Read the model definition and answer for the solid it produces. Units are mm, in the model's axes. Face numbers are marked on the shaded views. A direction names the side the tool comes from. Coordinates: 2 decimals unless noted, no trailing zeros. Order: outer loops, then holes, each group sorted by start corner. A loop starts at its lowest first (then second) coordinate and runs counter-clockwise, first axis right, second up. Notation, with made-up numbers: (61, 10.5) -> (112, 10.5) arc R28 ccw to (112, 38.5) -> close; hole circle Ø8 at (-37.5, 45). An arc over 180 degrees is marked (long way). Answer as a JSON object with one key per item and string values. Group by question number.
1) Determine the mould class of the marked faces 1, 2 and 3 for opening direction Z: released by +Z, released by -Z, zero draft, split by the parting line, or undercut.
2) A tool of negligible diameter and unlimited length cuts with its end or side. For the marked faces 4, 5, 6, 7 and 8, from which of +Z, -Z, +X, -X, +Y, -Y can it reach the whole face along a straight path? Write none if from no direction.
3) Section C-C on x = 104.5 is taken. Count the separate pieces of the cut face and the enclosed holes in it, and give its area (3 significant figures).
4) Section D-D on z = 31.5 is taken. Determine the outline of the cut face in (x, y), and give its area (3 significant figures).
5) Given pin 1 (3 mm diameter, centred on x = 87.5, z = 10.5, fed in from +Y); pin 2 (12 mm diameter, centred on y = 79, z = 19, fed in from -X); pin 3 (16.5 mm diameter, centred on y = 18.5, z = 22, fed in from -X), each flat-ended and moving along its own axis, determine where each tip first touches the part or whether it passes through.
6) Consider L1, parallel to Z at x = 105.5, y = 70.5; L2, parallel to Y at x = 118, z = 28.5; L3, parallel to Z at x = 96.5, y = 57. Determine where each line is inside the solid, lowest interval first.
7) Section B-B on y = 25 is taken. Determine the outline of the cut face in (x, z), and give its area (3 significant figures).
8) Section A-A on z = 7 is taken. Determine the outline of the cut face in (x, y), and give its area (3 significant figures).
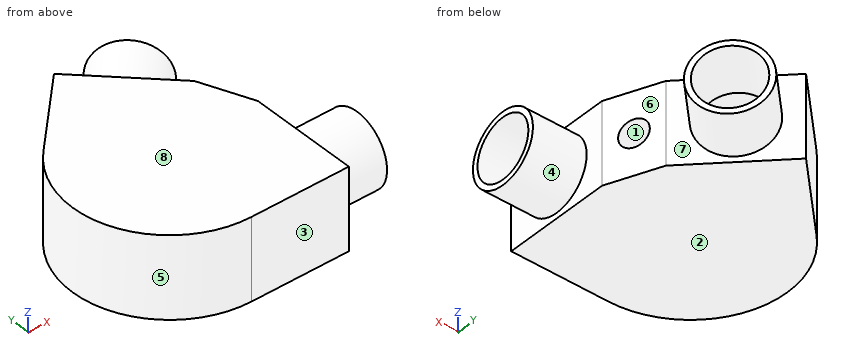
from build123d import *

# Parameters (mm, degrees)
F1_DEPTH = 38
F2_R     = 16.5
F3_DEPTH = 25
F4_R     = 45
F5_R     = 16.5
F6_DEPTH = 25
F7_R     = 6.35
F8_DEPTH = 50
F9_T     = -2.5


with BuildPart() as f1:
    # F0 (on Top) → F1 (new body)
    with BuildSketch(Plane.XY):
        Polygon((85.0829000017, 108.8944443027), (-23.811544301, 0), (130.188455699, 0), (130.188455699, 50), (120.4382390611, 73.5391052434), align=None)
    extrude(amount=F1_DEPTH)

    # F2 (on face) → F3 (join)
    with BuildSketch(Plane.YZ.offset(130.188455699)):
        with Locations((25, 19)):
            Circle(F2_R)
    extrude(amount=F3_DEPTH)

    # F4
    f4_edges = [f1.edges().sort_by_distance(p)[0] for p in [
        (-23.811544, 0, 19),
    ]]
    fillet(f4_edges, radius=F4_R)

    # F5 (on face) → F6 (join)
    with BuildSketch(Plane(origin=(96.9886721522, 96.9886721522, 0), x_dir=(-0.7071067812, 0.7071067812, 0), z_dir=(0.7071067812, 0.7071067812, 0))):
        with Locations((-8.1626955542, 19)):
            Circle(F5_R)
    extrude(amount=F6_DEPTH)

    # F7 (on face) → F8 (cut)
    with BuildSketch(Plane(origin=(128.8004673077, 53.3509003988, 0), x_dir=(-0.3826834324, 0.9238795325, 0), z_dir=(0.9238795325, 0.3826834324, 0))):
        with Locations((9.112283503, 19)):
            Circle(F7_R)
    extrude(amount=-F8_DEPTH, mode=Mode.SUBTRACT)

    # F9
    f9_openings = [f1.faces().sort_by_distance(p)[0] for p in [
        (155.188456, 25, 19),
        (120.438239, 108.894444, 19),
    ]]
    offset(amount=F9_T, openings=f9_openings, kind=Kind.INTERSECTION)


solid = f1.part
Worked answers:
{
 "1": {"face 1": "undercut", "face 2": "released by -Z", "face 3": "zero draft"},
 "2": {"face 4": "+X", "face 5": "+Z, -Z, -X", "face 6": "+Z, -Z, +X", "face 7": "none", "face 8": "+Z, +X, -X, +Y, -Y"},
 "3": {"separate pieces": "2", "enclosed holes": "2", "area": "867 mm²"},
 "4": {"outline": "(53.01, 76.82) arc R45 ccw to (84.83, 0) -> (130.19, 0) -> (130.19, 14.23) -> (155.19, 14.23) -> (155.19, 18.7) -> (127.69, 18.7) -> (127.69, 2.5) -> (84.83, 2.5) arc R42.5 cw to (54.78, 75.05) -> (85.08, 105.36) -> (96.53, 93.91) -> (115.98, 113.35) -> (112.82, 116.51) -> (95.14, 98.83) -> (85.08, 108.89) -> close; (105.45, 84.99) -> (118.32, 72.12) -> (127.69, 49.5) -> (127.69, 31.3) -> (155.19, 31.3) -> (155.19, 35.77) -> (130.19, 35.77) -> (130.19, 50) -> (120.44, 73.54) -> (110.38, 83.6) -> (128.05, 101.28) -> (124.9, 104.44) -> close", "area": "1,170 mm²"},
 "5": {"pin 1": "stops at y = 107.98", "pin 2": "stops at x = 49.6", "pin 3": "stops at x = 43.69"},
 "6": {"L1": "z = 0 to 2.5, 35.5 to 38", "L2": "y = 0 to 2.5, 72.44 to 75.98, 87.38 to 91.91", "L3": "z = 0 to 2.5, 13.13 to 24.87, 35.5 to 38"},
 "7": {"outline": "(44.52, 0) -> (130.19, 0) -> (130.19, 2.5) -> (155.19, 2.5) -> (155.19, 5) -> (127.69, 5) -> (127.69, 2.5) -> (47.33, 2.5) -> (47.33, 35.5) -> (127.69, 35.5) -> (127.69, 33) -> (155.19, 33) -> (155.19, 35.5) -> (130.19, 35.5) -> (130.19, 38) -> (44.52, 38) -> close", "area": "659 mm²"},
 "8": {"outline": "(53.01, 76.82) arc R45 ccw to (84.83, 0) -> (130.19, 0) -> (130.19, 13.68) -> (155.19, 13.68) -> (155.19, 17.79) -> (127.69, 17.79) -> (127.69, 2.5) -> (84.83, 2.5) arc R42.5 cw to (54.78, 75.05) -> (85.08, 105.36) -> (95.89, 94.55) -> (115.34, 113.99) -> (112.43, 116.9) -> (94.75, 99.22) -> (85.08, 108.89) -> close; (106.09, 84.35) -> (118.32, 72.12) -> (127.69, 49.5) -> (127.69, 32.21) -> (155.19, 32.21) -> (155.19, 36.32) -> (130.19, 36.32) -> (130.19, 50) -> (120.44, 73.54) -> (110.77, 83.21) -> (128.45, 100.89) -> (125.54, 103.8) -> close", "area": "1,120 mm²"}
}
